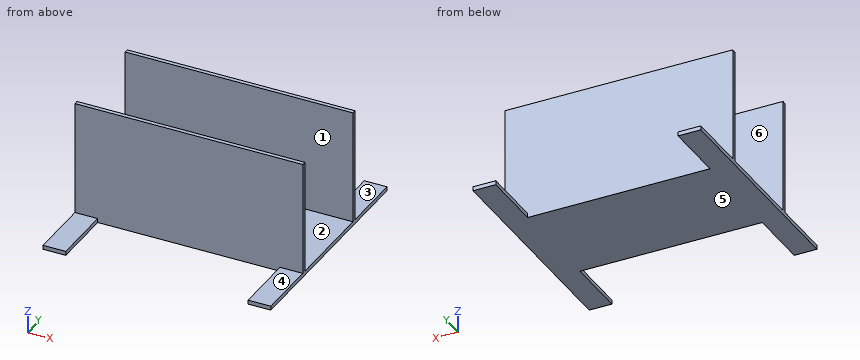
from build123d import *

# Parameters (mm, degrees)
F0_W          = 100
F0_H          = 45
F1_DEPTH      = 50
F1_DEPTH_BACK = 1.8
F2_T          = -1.8
F4_DEPTH      = 1.8


with BuildPart() as f1:
    # F0 (on Top) → F1 (new body, two sides)
    with BuildSketch(Plane.XY) as f1_sk:
        Rectangle(F0_W, F0_H)
    extrude(amount=F1_DEPTH)
    extrude(f1_sk.sketch, amount=-F1_DEPTH_BACK)

    # F2
    f2_openings = [f1.faces().sort_by_distance(p)[0] for p in [
        (0, 0, 50),
        (-50, 0, 24.1),
        (50, 0, 24.1),
    ]]
    offset(amount=F2_T, openings=f2_openings)

    # F3 (on Top) → F4 (join)
    with BuildSketch(Plane.XY):
        Polygon((-40, -50), (-40, 0), (-40, 50), (-50, 50), (-50, -50), align=None)
        Polygon((40, 50), (40, 0), (40, -50), (50, -50), (50, 50), align=None)
    extrude(amount=-F4_DEPTH)


solid = f1.part
Source: CAD feature listing. Evaluate the final solid. Frame: model axes, mm. Face numbers are marked on the shaded views. A direction names the side the tool comes from. Give positions to 0.01 mm unless a question says otherwise; leave off trailing zeros. Order: outer loops, then holes, each group sorted by start corner. A loop starts at its lowest first (then second) coordinate and runs counter-clockwise, first axis right, second up. Notation, with made-up numbers: (67.25, 85.25) -> (125.25, 85.25) arc R22 ccw to (125.25, 109.25) -> close; hole circle Ø2 at (31, -31.5). An arc over 180 degrees is marked (long way). Write item = value, one per line.
Item 1: Ray query, probe 1 along Y at (x, z) = (-9, 21); probe 2 along Z at (x, y) = (-11, -18). Return the intervals inside material, ascending.
Check result:
probe_1 = -22.5 to -20.7, 20.7 to 22.5
probe_2 = -1.8 to 0
Item 2: Section query A-A (z = 20.5). Output: boundary loops of the cut face in (x, y).
Check result:
outline = (-50, -22.5) -> (50, -22.5) -> (50, -20.7) -> (-50, -20.7) -> close; (-50, 20.7) -> (50, 20.7) -> (50, 22.5) -> (-50, 22.5) -> close
Item 3: Section query C-C (x = 1). Output: boundary loops of the cut face in (y, z), then the cut area to 3 significant figures.
Check result:
outline = (-22.5, -1.8) -> (22.5, -1.8) -> (22.5, 50) -> (20.7, 50) -> (20.7, 0) -> (-20.7, 0) -> (-20.7, 50) -> (-22.5, 50) -> close
area = 261 mm²
Item 4: Section query B-B (y = -32). Output: boundary loops of the cut face in (x, z), then the cut area to 3 significant figures.
Check result:
outline = (-50, -1.8) -> (-40, -1.8) -> (-40, 0) -> (-50, 0) -> close; (40, -1.8) -> (50, -1.8) -> (50, 0) -> (40, 0) -> close
area = 36.0 mm²
Item 5: Mould query, pull axis Y, two halves, no side actions, for the marked faces 1, 2 and 3. Classes: +Y half, -Y half, draft (parallel to the pull), parting line (faces both ways), or undercut.
Check result:
face_1 = undercut
face_2 = undercut
face_3 = draft
Item 6: Set-up query: the marked faces 4, 5 and 6. Return all of +Z, -Z, +X, -X, +Y, -Y with unobstructed straight access to the full face (end or side cutting, diameter ignored); none if empty.
Check result:
face_4 = +Z, +X, -X, -Y
face_5 = -Z, +X, -X, +Y, -Y
face_6 = +Z, +X, -X
Item 7: Contact query for flat-ended pins moving along their axis: pin 1 (3 mm diameter, centred on x = -46.5, y = -35, fed in from +Z); pin 2 (15 mm diameter, centred on x = 20, z = 21, fed in from +Y); pin 3 (1 mm diameter, centred on x = -38, y = -25.5, fed in from +Z); pin 4 (15.5 mm diameter, centred on x = -1.5, z = 36.5, fed in from -Y). Output: stop coordinate, or through.
Check result:
pin_1 = 0
pin_2 = 22.5
pin_3 = through
pin_4 = -22.5
Item 8: Section query D-D (x = 42.5). Output: boundary loops of the cut face in (y, z).
Check result:
outline = (-50, -1.8) -> (50, -1.8) -> (50, 0) -> (22.5, 0) -> (22.5, 50) -> (20.7, 50) -> (20.7, 0) -> (-20.7, 0) -> (-20.7, 50) -> (-22.5, 50) -> (-22.5, 0) -> (-50, 0) -> close
